from build123d import *

# Parameters (mm, degrees)
CYLINDER034_R               = 1.25
CYLINDER034_DEPTH           = 14
CYLINDER034_ROLL_ANGLE      = -89.999776
CYLINDER034_PITCH_ANGLE     = 1.4e-05
CYLINDER034_PLACEMENT_ANGLE = -9.999925
CYLINDER033_R               = 1.25
CYLINDER033_DEPTH           = 14
CYLINDER033_ROLL_ANGLE      = -89.999776
CYLINDER033_PITCH_ANGLE     = 1.4e-05
CYLINDER033_PLACEMENT_ANGLE = -9.999925
CYLINDER032_R               = 1.25
CYLINDER032_DEPTH           = 14
CYLINDER032_ROLL_ANGLE      = -89.999776
CYLINDER032_PITCH_ANGLE     = 1.4e-05
CYLINDER032_PLACEMENT_ANGLE = -9.999925
CYLINDER031_R               = 1.25
CYLINDER031_DEPTH           = 14
CYLINDER031_ROLL_ANGLE      = -89.999776
CYLINDER031_PITCH_ANGLE     = 1.4e-05
CYLINDER031_PLACEMENT_ANGLE = -9.999925
CYLINDER025_R               = 6.05
CYLINDER025_DEPTH           = 18
CYLINDER025_ROLL_ANGLE      = -89.999807
CYLINDER025_PITCH_ANGLE     = 8e-06
CYLINDER025_PLACEMENT_ANGLE = -9.999933
CYLINDER024_R               = 4.75
CYLINDER024_DEPTH           = 9
CYLINDER024_ROLL_ANGLE      = -89.999776
CYLINDER024_PITCH_ANGLE     = 1.4e-05
CYLINDER024_PLACEMENT_ANGLE = -9.999925
CYLINDER023_R               = 10
CYLINDER023_DEPTH           = 14
CYLINDER023_ROLL_ANGLE      = -89.999807
CYLINDER023_PITCH_ANGLE     = 8e-06
CYLINDER023_PLACEMENT_ANGLE = -9.999933


with BuildPart() as cylinder034:
    # Cylinder034 → Cylinder034 (new body)
    with BuildSketch(Plane.XY):
        Circle(CYLINDER034_R)
    extrude(amount=CYLINDER034_DEPTH)


with BuildPart() as cylinder034_1:
    # Cylinder034 roll: moved
    add(cylinder034.part.rotate(Axis((0, 0, 0), (1, 0, 0)), CYLINDER034_ROLL_ANGLE))


with BuildPart() as cylinder034_2:
    # Cylinder034 pitch: moved
    add(cylinder034_1.part.rotate(Axis((0, 0, 0), (0, 1, 0)), CYLINDER034_PITCH_ANGLE))


with BuildPart() as cylinder034_3:
    # Cylinder034 placement: moved
    add(cylinder034_2.part.moved(Location((39.936529, -25.15494, 7.500007))).rotate(Axis((39.936529, -25.15494, 7.500007), (0, 0, 1)), CYLINDER034_PLACEMENT_ANGLE))


with BuildPart() as cylinder033:
    # Cylinder033 → Cylinder033 (new body)
    with BuildSketch(Plane.XY):
        Circle(CYLINDER033_R)
    extrude(amount=CYLINDER033_DEPTH)


with BuildPart() as cylinder033_1:
    # Cylinder033 roll: moved
    add(cylinder033.part.rotate(Axis((0, 0, 0), (1, 0, 0)), CYLINDER033_ROLL_ANGLE))


with BuildPart() as cylinder033_2:
    # Cylinder033 pitch: moved
    add(cylinder033_1.part.rotate(Axis((0, 0, 0), (0, 1, 0)), CYLINDER033_PITCH_ANGLE))


with BuildPart() as cylinder033_3:
    # Cylinder033 placement: moved
    add(cylinder033_2.part.moved(Location((39.936521, -25.15501, 25.500007))).rotate(Axis((39.936521, -25.15501, 25.500007), (0, 0, 1)), CYLINDER033_PLACEMENT_ANGLE))


with BuildPart() as cylinder032:
    # Cylinder032 → Cylinder032 (new body)
    with BuildSketch(Plane.XY):
        Circle(CYLINDER032_R)
    extrude(amount=CYLINDER032_DEPTH)


with BuildPart() as cylinder032_1:
    # Cylinder032 roll: moved
    add(cylinder032.part.rotate(Axis((0, 0, 0), (1, 0, 0)), CYLINDER032_ROLL_ANGLE))


with BuildPart() as cylinder032_2:
    # Cylinder032 pitch: moved
    add(cylinder032_1.part.rotate(Axis((0, 0, 0), (0, 1, 0)), CYLINDER032_PITCH_ANGLE))


with BuildPart() as cylinder032_3:
    # Cylinder032 placement: moved
    add(cylinder032_2.part.moved(Location((32.058057, -23.765835, 25.500009))).rotate(Axis((32.058057, -23.765835, 25.500009), (0, 0, 1)), CYLINDER032_PLACEMENT_ANGLE))


with BuildPart() as cylinder031:
    # Cylinder031 → Cylinder031 (new body)
    with BuildSketch(Plane.XY):
        Circle(CYLINDER031_R)
    extrude(amount=CYLINDER031_DEPTH)


with BuildPart() as cylinder031_1:
    # Cylinder031 roll: moved
    add(cylinder031.part.rotate(Axis((0, 0, 0), (1, 0, 0)), CYLINDER031_ROLL_ANGLE))


with BuildPart() as cylinder031_2:
    # Cylinder031 pitch: moved
    add(cylinder031_1.part.rotate(Axis((0, 0, 0), (0, 1, 0)), CYLINDER031_PITCH_ANGLE))


with BuildPart() as cylinder031_3:
    # Cylinder031 placement: moved
    add(cylinder031_2.part.moved(Location((32.055183, -23.766017, 7.500006))).rotate(Axis((32.055183, -23.766017, 7.500006), (0, 0, 1)), CYLINDER031_PLACEMENT_ANGLE))


with BuildPart() as bohrung_lager:
    # Cylinder025 → Cylinder025 (new body)
    with BuildSketch(Plane.XY):
        Circle(CYLINDER025_R)
    extrude(amount=CYLINDER025_DEPTH)


with BuildPart() as bohrung_lager_1:
    # Cylinder025 roll: moved
    add(bohrung_lager.part.rotate(Axis((0, 0, 0), (1, 0, 0)), CYLINDER025_ROLL_ANGLE))


with BuildPart() as bohrung_lager_2:
    # Cylinder025 pitch: moved
    add(bohrung_lager_1.part.rotate(Axis((0, 0, 0), (0, 1, 0)), CYLINDER025_PITCH_ANGLE))


with BuildPart() as bohrung_lager_3:
    # Cylinder025 placement: moved
    add(bohrung_lager_2.part.moved(Location((35.652514, -26.433263, 16.499993))).rotate(Axis((35.652514, -26.433263, 16.499993), (0, 0, 1)), CYLINDER025_PLACEMENT_ANGLE))


with BuildPart() as cylinder024:
    # Cylinder024 → Cylinder024 (new body)
    with BuildSketch(Plane.XY):
        Circle(CYLINDER024_R)
    extrude(amount=CYLINDER024_DEPTH)


with BuildPart() as cylinder024_1:
    # Cylinder024 roll: moved
    add(cylinder024.part.rotate(Axis((0, 0, 0), (1, 0, 0)), CYLINDER024_ROLL_ANGLE))


with BuildPart() as cylinder024_2:
    # Cylinder024 pitch: moved
    add(cylinder024_1.part.rotate(Axis((0, 0, 0), (0, 1, 0)), CYLINDER024_PITCH_ANGLE))


with BuildPart() as cylinder024_3:
    # Cylinder024 placement: moved
    add(cylinder024_2.part.moved(Location((33.913531, -36.27808, 15.499961))).rotate(Axis((33.913531, -36.27808, 15.499961), (0, 0, 1)), CYLINDER024_PLACEMENT_ANGLE))


with BuildPart() as cut031:
    # Cylinder023 → Cylinder023 (new body)
    with BuildSketch(Plane.XY):
        Circle(CYLINDER023_R)
    extrude(amount=CYLINDER023_DEPTH)


with BuildPart() as cut031_1:
    # Cylinder023 roll: moved
    add(cut031.part.rotate(Axis((0, 0, 0), (1, 0, 0)), CYLINDER023_ROLL_ANGLE))


with BuildPart() as cut031_2:
    # Cylinder023 pitch: moved
    add(cut031_1.part.rotate(Axis((0, 0, 0), (0, 1, 0)), CYLINDER023_PITCH_ANGLE))


with BuildPart() as cut031_3:
    # Cylinder023 placement: moved
    add(cut031_2.part.moved(Location((35.652514, -26.433263, 16.499993))).rotate(Axis((35.652514, -26.433263, 16.499993), (0, 0, 1)), CYLINDER023_PLACEMENT_ANGLE))

    # Cut022: cut Cylinder024
    add(cylinder024_3.part, mode=Mode.SUBTRACT)

    # Cut023: cut bohrung_lager
    add(bohrung_lager_3.part, mode=Mode.SUBTRACT)

    # Cut028: cut Cylinder031
    add(cylinder031_3.part, mode=Mode.SUBTRACT)

    # Cut029: cut Cylinder032
    add(cylinder032_3.part, mode=Mode.SUBTRACT)

    # Cut030: cut Cylinder033
    add(cylinder033_3.part, mode=Mode.SUBTRACT)

    # Cut031: cut Cylinder034
    add(cylinder034_3.part, mode=Mode.SUBTRACT)


solid = cut031_3.part
Part model, mm, in its own coordinate system. Coordinates: 2 decimals unless noted, no trailing zeros.
(1) Pin check, flat tips, straight feed: pin 1 Ø6 at (x, z) = (37, 11.5) entering from -Y; pin 2 Ø10 at (x, z) = (33, 11.5) entering from -Y; pin 3 Ø5 at (y, z) = (-15, 20) entering from -X. Stop position of each tip, or through.
Check sheet entries:
pin 1: stops at y = -27.2
pin 2: stops at y = -26.84
pin 3: stops at x = 27.36
(2) Probe L1, parallel to Z at x = 42.75, y = -14.75; L2, parallel to X at y = -17.75, z = 21.5; L3, parallel to X at y = -18.5, z = 21. List the from-to ranges inside material, lowest first.
Check sheet entries:
L1: z = 8.3 to 13.04, 19.96 to 24.7
L2: x = 28.39 to 33.72, 40.64 to 45.98
L3: x = 27.98 to 32.95, 41.16 to 46.12
(3) Pull direction Z, two halves, no side cores. Call faces 1 (the face through (40.44, -19.24, 8.63)), 2 (the face through (35.569, -19.41, 6.585)): pulls with the +Z half, pulls with the -Z half, needs draft (parallel to the pull), parting line crosses it, or undercut.
Check sheet entries:
face 1: undercut
face 2: parting line crosses it
